Model file for the job. Use its own axes, mm. Give positions to 0.01 mm unless a question says otherwise; leave off trailing zeros. Loops run counter-clockwise (first coordinate to the right, second up) from the corner with the lowest first, then second, coordinate; pieces in that order, holes last. Notation, with made-up numbers: M -20,-35.75 L 39,-35.75 A18 ccw 39,-13.75 Z; hole C 76.25,-40 d5. An arc over 180 degrees is marked long. Use CSV: the item, a comma, the result in double quotes. Start each with the question number.
(1) Slice it at D-D on z = 213. List the corners of the cut face in (x, y), and give its area (3 significant figures).
(2) Slice it at C-C on y = 0. List the corners of the cut face in (x, z).
(3) Slice it at A-A on x = 0. List the corners of the cut face in (y, z), and give its area (3 significant figures).
(4) Slice it at B-B on z = 14. List the corners of the cut face in (x, y), and give its area (3 significant figures).
(5) Flat gauge pins, fed straight in: P1, Ø5, axis at x = 7.5, z = 69, coming from the +Y side; P2, Ø10, axis at y = 8.5, z = 102.5, coming from the -X side; P3, Ø3, axis at y = -2.5, z = 66.5, coming from the -X side. Where does each tip first touch, or does it go through?
(6) Wall check: line 1 along Y through (x, z) = (0, 235); line 2 along Y through (x, z) = (0, 33); line 3 along Z through (x, y) = (3, 5). Give the ranges that are in metal, low to high. Write a range as from..to.
```python
from build123d import *

# Parameters (mm, degrees)
SKETCH1_R               = 17.5
BOSS_EXTRUDE1_DEPTH     = 249
SKETCH2_R               = 6.5
CUT_EXTRUDE1_DEPTH      = 55
SKETCH9_R               = 10
CUT_EXTRUDE5_DEPTH      = 50
CUT_EXTRUDE6_DEPTH      = 251.226897035
CUT_EXTRUDE6_DEPTH_BACK = 251.226897035
SKETCH10_R              = 3


with BuildPart() as part:
    # Sketch1 → Boss-Extrude1 (new body)
    with BuildSketch(Plane.XY):
        Circle(SKETCH1_R)
    extrude(amount=BOSS_EXTRUDE1_DEPTH)

    # Sketch2 → Cut-Extrude1 (cut)
    with BuildSketch(Plane.XY.offset(249)):
        Circle(SKETCH2_R)
    extrude(amount=-CUT_EXTRUDE1_DEPTH, mode=Mode.SUBTRACT)

    # Sketch9 → Cut-Extrude5 (cut)
    with BuildSketch(Plane(origin=(0, 0, 0), x_dir=(-1, 0, 0), z_dir=(0, 0, -1))):
        Circle(SKETCH9_R)
    extrude(amount=-CUT_EXTRUDE5_DEPTH, mode=Mode.SUBTRACT)

    # Sketch10 → Cut-Extrude6 (cut, two sides: drawn at the far end of the back side and taken through both)
    with BuildSketch(Plane(origin=(0, 0, 0), x_dir=(1, 0, 0), z_dir=(0, 1, 0)).offset(-CUT_EXTRUDE6_DEPTH_BACK)):
        with Locations(Location((0, -14, 0), (0, 0, 270))):
            Circle(SKETCH10_R)
    extrude(amount=CUT_EXTRUDE6_DEPTH + CUT_EXTRUDE6_DEPTH_BACK, mode=Mode.SUBTRACT)


solid = part.part
```
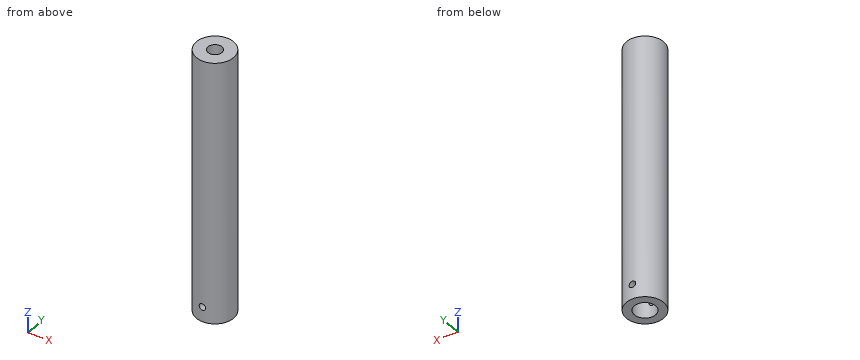
Reply:
1,outline,"C 0,0 d35; hole C 0,0 d13"
1,area,"829 mm^2"
2,outline,"M -17.5,0 L -10,0 L -10,50 L 10,50 L 10,0 L 17.5,0 L 17.5,249 L 6.5,249 L 6.5,194 L -6.5,194 L -6.5,249 L -17.5,249 Z"
3,outline,"M -17.5,0 L -10,0 L -10,11 L -17.5,11 Z; M -17.5,17 L -10,17 L -10,50 L 10,50 L 10,17 L 17.5,17 L 17.5,249 L 6.5,249 L 6.5,194 L -6.5,194 L -6.5,249 L -17.5,249 Z; M 10,0 L 17.5,0 L 17.5,11 L 10,11 Z"
3,area,"6,910 mm^2"
4,outline,"M -3,-17.24 L -3,-9.54 A10 cw -3,9.54 L -3,17.24 A17.5 ccw Z; M 3,-17.24 A17.5 ccw 3,17.24 L 3,9.54 A10 cw 3,-9.54 Z"
4,area,"557 mm^2"
5,P1,"stops at y = 16.77"
5,P2,"stops at x = -17.15"
5,P3,"stops at x = -17.47"
6,line 1,"y = -17.5..-6.5, 6.5..17.5"
6,line 2,"y = -17.5..-10, 10..17.5"
6,line 3,"z = 50..194"
